```python
from build123d import *

# Parameters (mm, degrees)
F0_W      = 177
F0_H      = 51
F0_R      = 3.3
F1_DEPTH  = 7.5
F2_DEPTH  = 1.5
F2_TAPER  = 6
F2_FACE_R = 3.1423436471
F3_DEPTH  = 7
F3_TAPER  = -5
F5_SIZE   = 1


# Not quite as in the source:
# - a fillet or chamfer that OpenCascade refuses, or shapes differently, is made with other operations: its cross-section is extruded or revolved along the edge and cut away or added


with BuildPart() as f1:
    # F0 (on Top) → F1 (new body)
    with BuildSketch(Plane.XY):
        with Locations((-21.5246523023, -20.9546978474)):
            Rectangle(F0_W, F0_H)
        with Locations((-90.5246523023, -19.9546978474)):
            Circle(F0_R, mode=Mode.SUBTRACT)
        with Locations((49.4753476977, -19.9546978474)):
            Circle(F0_R, mode=Mode.SUBTRACT)
        with Locations((-90.5246523023, -19.9546978474)):
            Circle(F0_R)
        with Locations((49.4753476977, -19.9546978474)):
            Circle(F0_R)
    extrude(amount=-F1_DEPTH)

    # F0 (on Top) → F2 (join)
    with BuildSketch(Plane.XY):
        with Locations((-90.5246523023, -19.9546978474)):
            Circle(F0_R)
        with Locations((49.4753476977, -19.9546978474)):
            Circle(F0_R)
    extrude(amount=F2_DEPTH, taper=F2_TAPER)

    # F2_face (on face) → F3 (join)
    with BuildSketch(Plane(origin=(49.4753476977, -19.9546978474, 1.5), x_dir=(1, 0, 0), z_dir=(0, 0, 1))):
        Circle(F2_FACE_R)
        with Locations((-140, 0)):
            Circle(F2_FACE_R)
    extrude(amount=F3_DEPTH, taper=F3_TAPER)

    # F4: chamfer of 0.6 on 2 edges, made by hand

    # F4_s1 → F4_t2 (revolve, cut)
    with BuildSketch(Plane.XZ.offset(19.9546978474)):
        Polygon((-86.8221814561, 7.9022831811), (-87.3698880105, 8.5), (-86.7698880105, 8.5), align=None)
    revolve(axis=Axis((-90.5246523023, -19.9546978474, 8.5), (0, 0, -1)), mode=Mode.SUBTRACT)

    # F4_s3 → F4_t4 (revolve, cut)
    with BuildSketch(Plane.XZ.offset(19.9546978474)):
        Polygon((53.1778185439, 7.9022831811), (52.6301119895, 8.5), (53.2301119895, 8.5), align=None)
    revolve(axis=Axis((49.4753476977, -19.9546978474, 8.5), (0, 0, -1)), mode=Mode.SUBTRACT)

    # F5
    f5_edges = [f1.edges().sort_by_distance(p)[0] for p in [
        (-110.024652, -20.954698, 0),
        (-21.524652, 4.545302, 0),
        (-21.524652, -46.454698, 0),
        (66.975348, -20.954698, 0),
        (-21.524652, 4.545302, -7.5),
        (-110.024652, -20.954698, -7.5),
        (-21.524652, -46.454698, -7.5),
        (66.975348, -20.954698, -7.5),
    ]]
    chamfer(f5_edges, length=F5_SIZE)


solid = f1.part
```
Design review of the part built by this model. Coordinates are the model's own, in mm. A direction names the side the tool comes from. Round coordinates to 2 decimals unless told otherwise and drop trailing zeros. Order: outer loops, then holes, each group sorted by start corner. A loop starts at its lowest first (then second) coordinate and runs counter-clockwise, first axis right, second up. Notation, with made-up numbers: M 18.25,64 L 66.25,64 A22 cw 66.25,73 Z; hole C 2.5,74 d2. An arc over 180 degrees is marked long. Put each result on its own line as item: value.
Q1. Consider section C-C (z = 3.75). State the section outline as (x, y) points.
Reported:
outline: C -90.52,-19.95 d6.68; C 49.48,-19.95 d6.68
Q2. Insertion check: pin 1 Ø14.5 at (x, y) = (-54, -19.5) entering from +Z. The pin has a flat end and moves straight along its axis. Give the tip position at first contact, or say it passes through.
Reported:
pin 1: z = 0
Q3. Draft analysis for pull direction X (two halves, no side actions). For faces 1 (the face through (-23, 4.545, -4)), 2 (the face through (-110.025, -21, -4)), 3 (the face through (46.756, -22.04, 4.746)), 4 (the face through (47.13, -17.8, 1.09)), state which applies: released by +X, released by -X, zero draft, split by the parting line, or undercut.
Reported:
face 1: zero draft
face 2: released by -X
face 3: undercut
face 4: undercut
Q4. Consider section B-B (y = -38). State the section outline as (x, z) points.
Reported:
outline: M -110.02,-6.5 L -109.02,-7.5 L 65.98,-7.5 L 66.98,-6.5 L 66.98,-1 L 65.98,0 L -109.02,0 L -110.02,-1 Z
Q5. Machinability: for faces 5 (the face through (-23, -21, -7.5)), 6 (the face through (-93.707, -19.815, 1.094)), which of the approach directions +Z, -Z, +X, -X, +Y, -Y give a long, thin tool a straight path to every point of the face, cutting with its end or side? Answer none if there is none.
Reported:
face 5: -Z, +X, -X, +Y, -Y
face 6: none
Q6. To check wall thickness, follow line 1 (Z direction, x = -74, y = -1.5); line 2 (X direction, y = -11, z = -0.5); line 3 (Y direction, x = -27.5, z = -0.75). State the ranges of each line that lie inside material, in increasing order.
Reported:
line 1: -7.5 to 0
line 2: -109.52 to 66.48
line 3: -46.2 to 4.3
Q7. Consider section A-A (x = -80). State the section outline as (y, z) points.
Reported:
outline: M -46.45,-6.5 L -45.45,-7.5 L 3.55,-7.5 L 4.55,-6.5 L 4.55,-1 L 3.55,0 L -45.45,0 L -46.45,-1 Z
